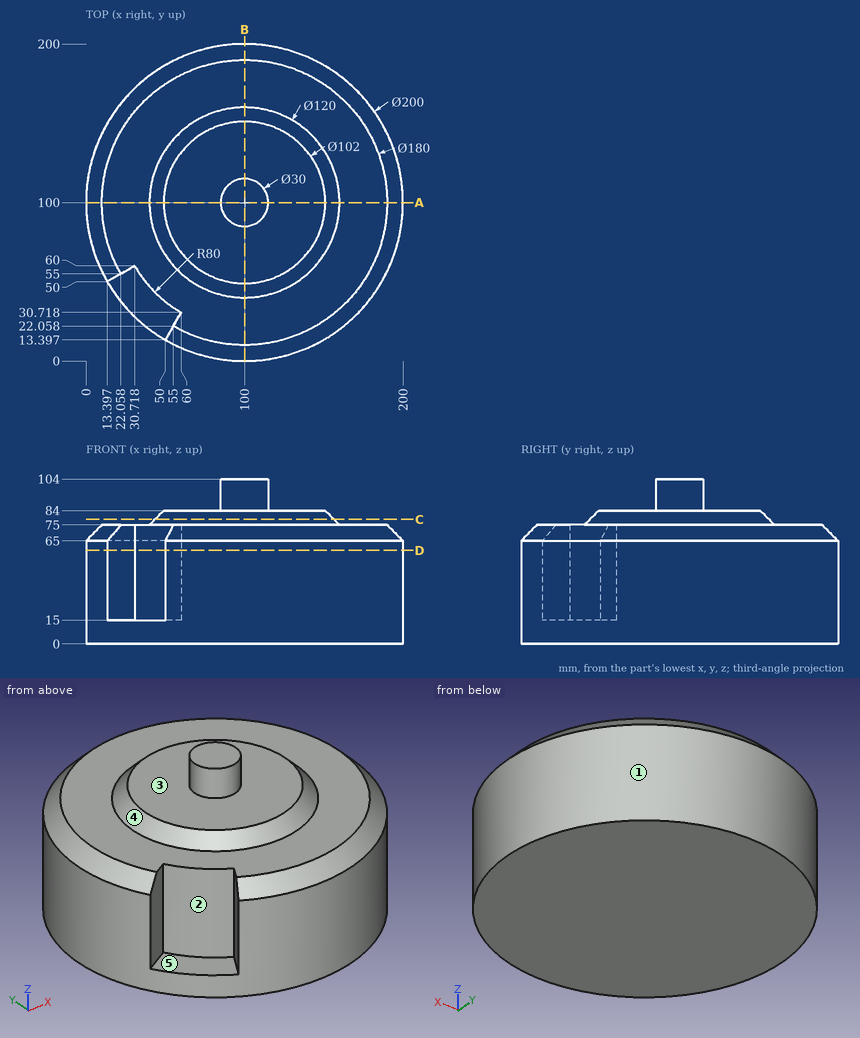
Could you check a few things on this drawing? It's one solid part, dimensions in mm from its lowest x, y, z. A direction names the side the tool comes from. Coordinates: 2 decimals unless noted, no trailing zeros. Order: outer loops, then holes, each group sorted by start corner. A loop starts at its lowest first (then second) coordinate and runs counter-clockwise, first axis right, second up.
1. If we section it at C-C (z = 78.5): Please give me the cut outline in (x, y).
2. If we section it at D-D (z = 59): Please give me the cut outline in (x, y).
3. Thinking about a two-plate mould opening in X: for the marked faces 3, 4 and 5, which applies, +X half, -X half, draft (parallel to the pull), parting line (faces both ways), or undercut?
4. If we section it at A-A (y = 100): Please give me the cut outline in (x, z).
5. For the marked faces 1 and 2, which set-ups out of +Z, -Z, +X, -X, +Y, -Y let a thin tool reach every point of the face, with its end or its side?
6. I need wall thicknesses on line 1 (Z direction, x = 128, y = 20); line 2 (X direction, y = 97, z = 46.5) (1 decimal); line 3 (Z direction, x = 135, y = 69.5). Which ranges of each line are inside material? Lowest first, please.
7. I'm going to push flat-ended pins straight in: pin 1 (14 mm diameter, centred on x = 37, y = 41, fed in from +Z); pin 2 (8 mm diameter, centred on x = 47, y = 77, fed in from +Z) (1 decimal); pin 3 (3 mm diameter, centred on x = 80, z = 33.5, fed in from +Y). Where does each tip first touch, or does it pass through?
Entries:
1. outline: circle Ø113 at (100, 100)
2. outline: (13.4, 50) - (30.72, 60) arc R80 ccw to (60, 30.72) - (50, 13.4) arc R100 ccw (long way) to start
3. face 3: draft
3. face 4: parting line
3. face 5: undercut
4. outline: (0, 0) - (200, 0) - (200, 65) - (190, 75) - (160, 75) - (151, 84) - (115, 84) - (115, 104) - (85, 104) - (85, 84) - (49, 84) - (40, 75) - (10, 75) - (0, 65) - close
5. face 1: +Z, -Z
5. face 2: +Z
6. line 1: z = 0 to 75
6. line 2: x = 0 to 200
6. line 3: z = 0 to 84
7. pin 1: stops at z = 75
7. pin 2: stops at z = 81.2
7. pin 3: stops at y = 198.27
